Here's how the part is built. I have some questions about the finished solid (model axes, mm). A direction names the side the tool comes from. Coordinates: 2 decimals unless noted, no trailing zeros. Loops run counter-clockwise (first coordinate to the right, second up) from the corner with the lowest first, then second, coordinate; pieces in that order, holes last. Notation, with made-up numbers: (11.25, -32.75) -> (63.25, -32.75) arc R11 ccw to (63.25, -22.75) -> close; hole circle Ø1 at (50, -28.5). An arc over 180 degrees is marked (long way). Answer as a JSON object with one key per item and string values. Group by question number.
Q1. On a 3-axis mill with a long thin cutter (end or side, diameter ignored), from which of +Z, -Z, +X, -X, +Y, -Y can I reach the whole of each face in a straight line? I mean faces 1 (the flat face through (-32, -1, -1)), 2 (the flat face through (-1, 0, 1)). Say none if no direction works.
Q2. I want a section at B-B on y = -1.2. Write out the boundary of the cut face in (x, z), then the cut area to 3 significant figures.
Q3. Thinking about a two-plate mould opening in Z: for faces 3 (the flat face through (-24.171, -1, 0)), 4 (the flat face through (-1, -3, 1)), which applies, released by +Z, released by -Z, zero draft, split by the parting line, or undercut?
Q4. I'm going to push flat-ended pins straight in: pin 1 (0.6 mm diameter, centred on y = -1.5, z = 0.5, fed in from -X); pin 2 (5 mm diameter, centred on x = 22.5, z = -25, fed in from +Y); pin 3 (0.9 mm diameter, centred on x = -36, y = -2, fed in from +Z). Where does each tip first touch, or does it pass through?
Q5. I want a section at A-A on x = 14. Write out the boundary of the cut face in (y, z).
Q6. I need wall thicknesses on line 1 (Z direction, x = -1, y = -0.35); line 2 (X direction, y = -1.9, z = 28); line 3 (Z direction, x = 25, y = -0.95). Which ranges of each line are inside material? Lowest first, please.
```python
from build123d import *

# Parameters (mm, degrees)
F0_R     = 40
F1_DEPTH = 3
F2_W     = 33.162359
F2_H     = 1
F3_DEPTH = 24.9
F4_DEPTH = 25


with BuildPart() as f1:
    # F0 (on Front) → F1 (new body)
    with BuildSketch(Plane.XZ):
        Circle(F0_R)
    extrude(amount=F1_DEPTH)

    # F2 (on Front) → F3 (cut)
    with BuildSketch(Plane.XZ):
        with Locations((-40.752544, 0.5)):
            Rectangle(F2_W, F2_H)
    extrude(amount=F3_DEPTH, mode=Mode.SUBTRACT)

    # F2 (on Front) → F4 (cut)
    with BuildSketch(Plane.XZ):
        with Locations((-40.752544, 0.5)):
            Rectangle(F2_W, F2_H)
        with Locations((-40.752544, -0.5)):
            Rectangle(F2_W, F2_H)
    extrude(amount=F4_DEPTH, mode=Mode.SUBTRACT)


solid = f1.part
```
Result set:
{
 "1": {"face 1": "-X, +Y, -Y", "face 2": "+Z, -Z, +X, -X, +Y"},
 "2": {"outline": "(-39.99, -1) arc R40 ccw (long way) to (-39.99, 1) -> (-24.17, 1) -> (-24.17, -1) -> close", "area": "4,990 mm²"},
 "3": {"face 3": "undercut", "face 4": "zero draft"},
 "4": {"pin 1": "stops at x = -24.17", "pin 2": "stops at y = 0", "pin 3": "stops at z = 18.34"},
 "5": {"outline": "(-3, -37.47) -> (0, -37.47) -> (0, 37.47) -> (-3, 37.47) -> close"},
 "6": {"line 1": "z = -39.99 to 39.99", "line 2": "x = -28.57 to 28.57", "line 3": "z = -31.22 to 31.22"}
}
